Part print with two shaded views. Sizes in mm from the minimum x, y, z corner. Coordinates: 2 decimals unless noted, no trailing zeros. Write each loop counter-clockwise with the first axis right and the second up, starting at its lowest first coordinate (ties: lowest second). Pieces come first, ordered by that corner, then holes.
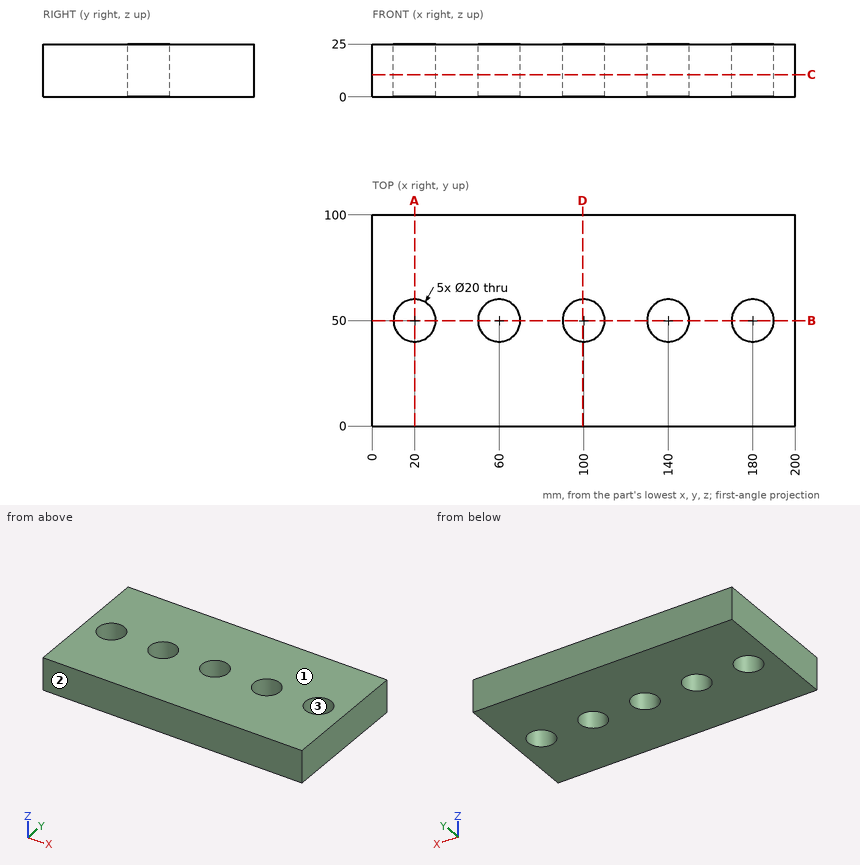
(1) Flat gauge pin, fed straight in: P1, Ø18, axis at x = 180, y = 50, coming from the -Z side. Where does the tip first touch, or does it go through?
(2) Slice it at C-C, the plane z = 10.5. List the corners of the cut face in (x, y), and give its area (3 significant figures).
(3) Two-plate mould, pull along Y, no slides. Class the marked faces 1, 2 and 3: pulls with the +Y half, pulls with the -Y half, needs draft (parallel to the pull), parting line crosses it, or undercut.
(4) Slice it at A-A, the plane x = 20. List the corners of the cut face in (y, z), and give its area (3 significant figures).
(5) Probe L1, parallel to X at y = 50, z = 18.5; L2, parallel to X at y = 58.5, z = 1.25; L3, parallel to Y at x = 20, z = 19.5. List the from-to ranges inside material, lowest first.
(6) Slice it at D-D, the plane x = 99.5. List the corners of the cut face in (y, z).
(7) Slice it at B-B, the plane y = 50. List the corners of the cut face in (x, z), and give its area (3 significant figures).
Results:
1. P1: passes through
2. outline: (0, 0) - (200, 0) - (200, 100) - (0, 100) - close; hole circle Ø20 at (20, 50); hole circle Ø20 at (60, 50); hole circle Ø20 at (100, 50); hole circle Ø20 at (140, 50); hole circle Ø20 at (180, 50)
2. area: 18,400 mm2
3. face 1: needs draft
3. face 2: pulls with the -Y half
3. face 3: undercut
4. outline: (0, 0) - (40, 0) - (40, 25) - (0, 25) - close; (60, 0) - (100, 0) - (100, 25) - (60, 25) - close
4. area: 2,000 mm2
5. L1: x = 0 to 10, 30 to 50, 70 to 90, 110 to 130, 150 to 170, 190 to 200
5. L2: x = 0 to 14.73, 25.27 to 54.73, 65.27 to 94.73, 105.27 to 134.73, 145.27 to 174.73, 185.27 to 200
5. L3: y = 0 to 40, 60 to 100
6. outline: (0, 0) - (40.01, 0) - (40.01, 25) - (0, 25) - close; (59.99, 0) - (100, 0) - (100, 25) - (59.99, 25) - close
7. outline: (0, 0) - (10, 0) - (10, 25) - (0, 25) - close; (30, 0) - (50, 0) - (50, 25) - (30, 25) - close; (70, 0) - (90, 0) - (90, 25) - (70, 25) - close; (110, 0) - (130, 0) - (130, 25) - (110, 25) - close; (150, 0) - (170, 0) - (170, 25) - (150, 25) - close; (190, 0) - (200, 0) - (200, 25) - (190, 25) - close
7. area: 2,500 mm2
